from build123d import *

# Parameters (mm, degrees)
SKETCH1_W                    = 60
SKETCH1_H                    = 60
SKETCH1_R                    = 20
BOSS_EXTRUDE1_DEPTH          = 3.5
SKETCH2_R                    = 20
BOSS_EXTRUDE2_DEPTH          = 4
F_5_0_5_DIAMETER_HOLE1_D     = 5
F_5_0_5_DIAMETER_HOLE1_DEPTH = 25
F_5_0_5_DIAMETER_HOLE1_TIP   = 1.502151548


with BuildPart() as part:
    # Sketch1 → Boss-Extrude1 (new body)
    with BuildSketch(Plane(origin=(0, 0, 0), x_dir=(1, 0, 0), z_dir=(0, 1, 0))):
        Rectangle(SKETCH1_W, SKETCH1_H)
        Circle(SKETCH1_R, mode=Mode.SUBTRACT)
    extrude(amount=BOSS_EXTRUDE1_DEPTH)

    # Sketch2 → Boss-Extrude2 (add)
    with BuildSketch(Plane(origin=(0, 3.5, -3.5), x_dir=(1, 0, 0), z_dir=(0, -1, 0))):
        with BuildLine():
            Line((45, -26.5), (-45, -26.5))
            ThreePointArc((-45, -26.5), (-52.071067812, -23.571067812), (-55, -16.5))
            Line((-55, -16.5), (-55, 23.5))
            ThreePointArc((-55, 23.5), (-52.071067812, 30.571067812), (-45, 33.5))
            Line((-45, 33.5), (45, 33.5))
            ThreePointArc((45, 33.5), (52.071067812, 30.571067812), (55, 23.5))
            Line((55, 23.5), (55, -16.5))
            ThreePointArc((55, -16.5), (52.071067812, -23.571067812), (45, -26.5))
        make_face()
        with Locations((0, 3.5)):
            Circle(SKETCH2_R, mode=Mode.SUBTRACT)
        with BuildLine():
            Line((-47, -15), (-47, -18))
            ThreePointArc((-47, -18), (-45, -20), (-43, -18))
            Line((-43, -18), (-43, -15))
            ThreePointArc((-43, -15), (-45, -13), (-47, -15))
        make_face(mode=Mode.SUBTRACT)
        with BuildLine():
            Line((-43, 25), (-43, 22))
            ThreePointArc((-43, 22), (-45, 20), (-47, 22))
            Line((-47, 22), (-47, 25))
            ThreePointArc((-47, 25), (-45, 27), (-43, 25))
        make_face(mode=Mode.SUBTRACT)
        with BuildLine():
            Line((43, -18), (43, -15))
            ThreePointArc((43, -15), (45, -13), (47, -15))
            Line((47, -15), (47, -18))
            ThreePointArc((47, -18), (45, -20), (43, -18))
        make_face(mode=Mode.SUBTRACT)
        with BuildLine():
            Line((47, 22), (47, 25))
            ThreePointArc((47, 25), (45, 27), (43, 25))
            Line((43, 25), (43, 22))
            ThreePointArc((43, 22), (45, 20), (47, 22))
        make_face(mode=Mode.SUBTRACT)
    extrude(amount=-BOSS_EXTRUDE2_DEPTH)

    # Ø5.0 (5) Diameter Hole1
    with Locations(Plane(origin=(233.298234679, 0, -449.602484579), x_dir=(-1, 0, 0), z_dir=(0, -1, 0))):
        with Locations((256.868234679, -473.172484579), (209.728234679, -473.172484579), (209.728234679, -426.032484579), (256.868234679, -426.032484579)):
            Hole(F_5_0_5_DIAMETER_HOLE1_D / 2, depth=F_5_0_5_DIAMETER_HOLE1_DEPTH)
            with Locations((0, 0, -(F_5_0_5_DIAMETER_HOLE1_DEPTH + F_5_0_5_DIAMETER_HOLE1_TIP / 2))):  # 118° drill point
                Cone(0, F_5_0_5_DIAMETER_HOLE1_D / 2, F_5_0_5_DIAMETER_HOLE1_TIP, mode=Mode.SUBTRACT)


solid = part.part
The listing builds one solid part. Answer for the finished solid, in the listing's coordinates (mm). A direction names the side the tool comes from. Round coordinates to 2 decimals unless told otherwise and drop trailing zeros. Order: outer loops, then holes, each group sorted by start corner. A loop starts at its lowest first (then second) coordinate and runs counter-clockwise, first axis right, second up. Notation, with made-up numbers: (23.25, 35.25) -> (37.25, 35.25) arc R18 cw to (37.25, 54.25) -> close; hole circle Ø9 at (29.5, -0.75). An arc over 180 degrees is marked (long way). Write each question's results on one line, items separated by ' | '. Start each with the question number.
Q1. Find section B-B (y = 1.25). Determine the outline of the cut face in (x, z).
Q2. Straight lines are drawn through the part: probe 1 along Z at (x, y) = (-23.57, 5.75); probe 2 along Z at (x, y) = (0, 4.75); probe 3 along X at (y, z) = (3.75, 0). For each, find the intervals that lie inside material, in ascending order. Write a range as from..to.
Q3. Find section D-D (x = -40.5). Determine the outline of the cut face in (y, z).
Q4. Find section C-C (y = 6.25). Give the number of separate pieces and of enclosed holes in the cut face, then the cut area to 3 significant figures.
Q5. Which of the six approach directions +Z, -Z, +X, -X, +Y, -Y give full straight-line access (tool end or side, diameter ignored) to faces 1 (the flat face through (-42, 3.5, 0)), 2 (the cylindrical face through (-45, 5.5, -16.5)), 3 (the flat face through (30, 2, 0))?
Q6. The mould has two halves that part along X. Classify faces 4 (the cylindrical face through (-51.99, 5.47, -27.15)), 5 (the cylindrical face through (45, 5.5, -23.5)), 6 (the flat face through (-1, 4, 30)): pulls with the +X half, pulls with the -X half, needs draft (parallel to the pull), parting line crosses it, or undercut.
Q7. Each of these flat-tipped pins is pushed along its axis until it touches: pin 1 (6.5 mm diameter, centred on x = -23.57, z = 23.57, fed in from -Y); pin 2 (4.5 mm diameter, centred on x = 23.57, z = 23.57, fed in from -Y); pin 3 (7.5 mm diameter, centred on x = 46.5, z = -2, fed in from -Y); pin 4 (1 mm diameter, centred on y = 1.5, z = 11, fed in from +X). Where does it stop, or does it pass through?
Q8. Find section A-A (z = 0). Determine the outline of the cut face in (x, y).
Worked answers:
1) outline: (-30, -30) -> (30, -30) -> (30, 30) -> (-30, 30) -> close; hole circle Ø5 at (-23.57, -23.57); hole circle Ø5 at (-23.57, 23.57); hole circle Ø40 at (0, 0); hole circle Ø5 at (23.57, -23.57); hole circle Ø5 at (23.57, 23.57)
2) probe 1: z = -30..-26.07, -21.07..21.07, 26.07..30 | probe 2: z = -30..-20, 20..30 | probe 3: x = -55..-20, 20..55
3) outline: (3.5, -30) -> (7.5, -30) -> (7.5, 30) -> (3.5, 30) -> close
4) separate pieces: 1 | enclosed holes: 9 | area: 5,080 mm2
5) face 1: +Z, -Z, -X, -Y | face 2: +Y, -Y | face 3: +Z, -Z, +X, -Y
6) face 4: pulls with the -X half | face 5: undercut | face 6: needs draft
7) pin 1: stops at y = 0 | pin 2: passes through | pin 3: stops at y = 3.5 | pin 4: stops at x = 30
8) outline: (-55, 3.5) -> (-30, 3.5) -> (-30, 0) -> (-20, 0) -> (-20, 7.5) -> (-55, 7.5) -> close; (20, 0) -> (30, 0) -> (30, 3.5) -> (55, 3.5) -> (55, 7.5) -> (20, 7.5) -> close
